from build123d import *

# Parameters (mm, degrees)
SKETCH003_R             = 62
SKETCH003_R_2           = 1.8
PAD002_DEPTH            = 3
SKETCH005_R             = 5
PAD004_DEPTH            = 28
SKETCH011_R             = 1.8
POCKET004_DEPTH         = 3
PAD011_DEPTH            = 5
PAD012_DEPTH            = 5
SKETCH007_R             = 1.5
POCKET002_DEPTH         = 15
BODY001_PLACEMENT_ANGLE = 180


with BuildPart() as part:
    # Sketch003 → Pad002 (new body)
    with BuildSketch(Plane.XY):
        Circle(SKETCH003_R)
        with Locations((8.485281, 8.485281)):
            Circle(SKETCH003_R_2, mode=Mode.SUBTRACT)
        with Locations((-8.485281, 8.485281)):
            Circle(SKETCH003_R_2, mode=Mode.SUBTRACT)
        with Locations((-8.485281, -8.485281)):
            Circle(SKETCH003_R_2, mode=Mode.SUBTRACT)
        with Locations((8.485281, -8.485281)):
            Circle(SKETCH003_R_2, mode=Mode.SUBTRACT)
    extrude(amount=PAD002_DEPTH)

    # Sketch005 → Pad004 (join)
    with BuildSketch(Plane.XY):
        with Locations((33.234019, 33.234019)):
            Circle(SKETCH005_R)
        with Locations((-33.234019, 33.234019)):
            Circle(SKETCH005_R)
        with Locations((-33.234019, -33.234019)):
            Circle(SKETCH005_R)
        with Locations((33.234019, -33.234019)):
            Circle(SKETCH005_R)
    extrude(amount=PAD004_DEPTH)

    # Sketch011 → Pocket004 (cut, symmetric)
    with BuildSketch(Plane.XY):
        with Locations((27.5, 47.631397)):
            Circle(SKETCH011_R)
        with Locations((-47.631397, 27.5)):
            Circle(SKETCH011_R)
        with Locations((-27.5, -47.631397)):
            Circle(SKETCH011_R)
        with Locations((47.631397, -27.5)):
            Circle(SKETCH011_R)
        with Locations((-27.5, 47.631397)):
            Circle(SKETCH011_R)
        with Locations((47.631397, 27.5)):
            Circle(SKETCH011_R)
        with Locations((27.5, -47.631397)):
            Circle(SKETCH011_R)
        with Locations((-47.631397, -27.5)):
            Circle(SKETCH011_R)
    extrude(amount=POCKET004_DEPTH, both=True, mode=Mode.SUBTRACT)

    # Sketch018 → Pad011 (join, symmetric)
    with BuildSketch(Plane(origin=(0, 0, 0), x_dir=(-0.707107, 0.707107, 0), z_dir=(0.707107, 0.707107, 0))):
        with BuildLine():
            Line((-47, 28), (-47, 3))
            Line((-47, 3), (-27, 3))
            ThreePointArc((-42, 18), (-37.606602, 7.393398), (-27, 3))
            Line((-42, 18), (-42, 28))
            Line((-42, 28), (-47, 28))
        make_face()
        with BuildLine():
            Line((47, 28), (47, 3))
            Line((47, 3), (27, 3))
            ThreePointArc((27, 3), (37.606602, 7.393398), (42, 18))
            Line((42, 18), (42, 28))
            Line((42, 28), (47, 28))
        make_face()
    extrude(amount=PAD011_DEPTH, both=True)

    # Sketch019 → Pad012 (join, symmetric)
    with BuildSketch(Plane(origin=(0, 0, 0), x_dir=(0.707107, 0.707107, 0), z_dir=(0.707107, -0.707107, 0))):
        with BuildLine():
            Line((-47, 28), (-47, 3))
            Line((-47, 3), (-27, 3))
            ThreePointArc((-42, 18), (-37.606602, 7.393398), (-27, 3))
            Line((-42, 18), (-42, 28))
            Line((-42, 28), (-47, 28))
        make_face()
        with BuildLine():
            Line((47, 28), (47, 3))
            Line((47, 3), (27, 3))
            ThreePointArc((27, 3), (37.606602, 7.393398), (42, 18))
            Line((42, 18), (42, 28))
            Line((42, 28), (47, 28))
        make_face()
    extrude(amount=PAD012_DEPTH, both=True)

    # Sketch007 → Pocket002 (cut)
    with BuildSketch(Plane.XY.offset(28)):
        with Locations((33.234019, 33.234019)):
            Circle(SKETCH007_R)
        with Locations((-33.234019, 33.234019)):
            Circle(SKETCH007_R)
        with Locations((-33.234019, -33.234019)):
            Circle(SKETCH007_R)
        with Locations((33.234019, -33.234019)):
            Circle(SKETCH007_R)
    extrude(amount=-POCKET002_DEPTH, mode=Mode.SUBTRACT)


with BuildPart() as part_1:
    # Body001 placement: moved
    add(part.part.moved(Location((0, 0, 25))).rotate(Axis((0, 0, 25), (0, 0, -1)), BODY001_PLACEMENT_ANGLE))


solid = part_1.part
Model file for the job. Use its own axes, mm. A direction names the side the tool comes from. Give positions to 0.01 mm unless a question says otherwise; leave off trailing zeros. Loops run counter-clockwise (first coordinate to the right, second up) from the corner with the lowest first, then second, coordinate; pieces in that order, holes last.
1) Wall check: line 1 (Y direction, x = -34, z = 44.25) (3 decimals); line 2 (Z direction, x = 22.5, y = 31); line 3 (Y direction, x = -35.5, z = 29.25). Give the ranges that are in metal, low to high.
2) Pull direction Y, two halves, no side cores. Call faces 6 (the cylindrical face through (49.43, 27.42, 26.52)), 7 (the flat face through (1, -1, 25)), 8 (the flat face through (-26.85, -33.92, 37.78)), 9 (the flat face through (-33.92, 26.85, 37.78)): +Y half, -Y half, draft (parallel to the pull), parting line (faces both ways), or undercut.
3) Flat gauge pins, fed straight in: pin 1 Ø3 at (y, z) = (32, 45.5) entering from +X; pin 2 Ø2.5 at (x, y) = (-33.23, 33.23) entering from +Z; pin 3 Ø4 at (x, y) = (47.63, -27.5) entering from +Z; pin 4 Ø3 at (x, y) = (-27.5, 47.63) entering from -Z. Where does each tip first touch, or does it go through?
4) Saw through at D-D (y = 0). Write the cut outline in (x, z).
5) Saw through at B-B (z = 30.25). Write the cut outline in (x, y).
6) Tool access for faces 1 (the flat face through (26.85, 33.92, 37.78)), 2 (the flat face through (33.92, 26.85, 37.78)), 3 (the cylindrical face through (36.85, 36.69, 40.33)), 4 (the flat face through (-32, 32, 53)), 5 (the cylindrical face through (-28.331, -46.034, 26.479)): list every direction of +Z, -Z, +X, -X, +Y, -Y with a clear straight run to the whole face (end or side of a thin tool).
Answer block:
1. line 1: y = -38.175 to -34.524, -31.944 to -26.929, 26.929 to 31.944, 34.524 to 38.175
1. line 2: z = 25 to 28
1. line 3: y = -37.69 to -28.43, 28.43 to 37.69
2. face 6: undercut
2. face 7: draft
2. face 8: -Y half
2. face 9: undercut
3. pin 1: stops at x = 38.23
3. pin 2: stops at z = 38
3. pin 3: stops at z = 28
3. pin 4: passes through
4. outline: (-62, 25) - (62, 25) - (62, 28) - (-62, 28) - close
5. outline: (-36.77, -29.7) arc R5 ccw to (-29.7, -36.77) - (-21.14, -28.21) - (-28.21, -21.14) - close; (-36.77, 29.7) - (-28.21, 21.14) - (-21.14, 28.21) - (-29.7, 36.77) arc R5 ccw to start; (21.14, -28.21) - (29.7, -36.77) arc R5 ccw to (36.77, -29.7) - (28.21, -21.14) - close; (21.14, 28.21) - (28.21, 21.14) - (36.77, 29.7) arc R5 ccw to (29.7, 36.77) - close
6. face 1: +Z, +Y
6. face 2: +Z, +X
6. face 3: +Z
6. face 4: +Z, +X, -X, +Y, -Y
6. face 5: +Z, -Z
